The drawing under review shows one solid part. Ordinate dimensions are in mm from its lowest x, y, z. Round coordinates to 2 decimals unless told otherwise and drop trailing zeros. Order: outer loops, then holes, each group sorted by start corner. A loop starts at its lowest first (then second) coordinate and runs counter-clockwise, first axis right, second up. Notation, with made-up numbers: M 78.5,36.25 L 136.5,36.25 A19 ccw 136.5,51.25 Z; hole C 27,-35 d5. An arc over 180 degrees is marked long. Answer as a JSON object with one key per item and string values.
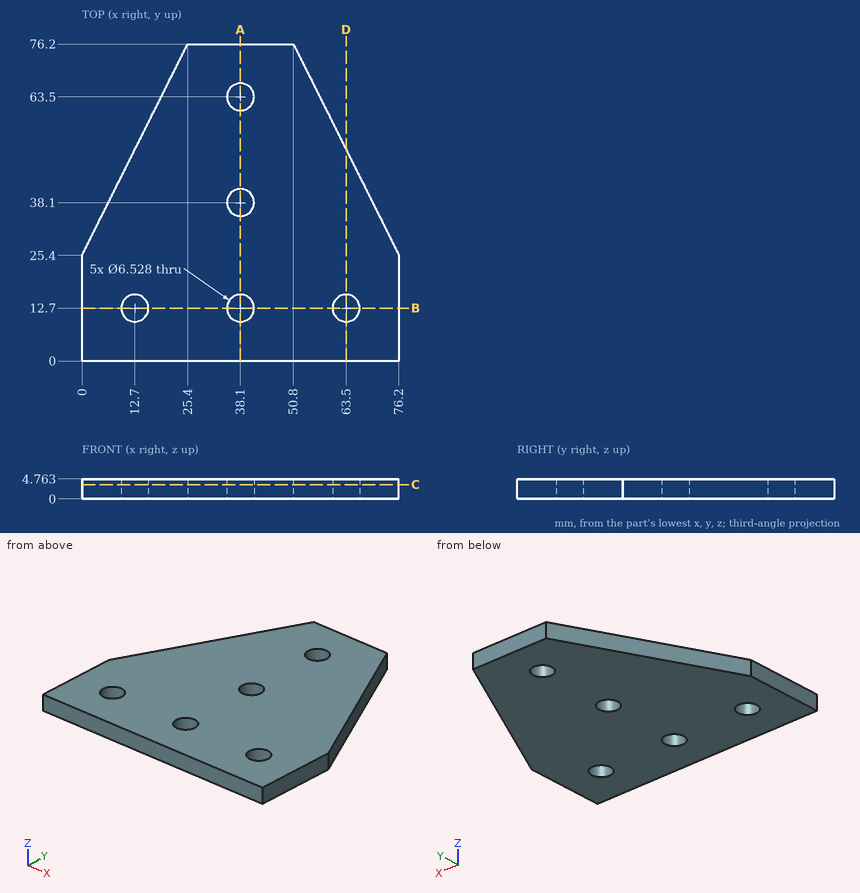
1) Add section A-A on x = 38.1. State the section outline as (y, z) points.
Geometry check:
{"outline": "M 0,0 L 9.44,0 L 9.44,4.76 L 0,4.76 Z; M 15.96,0 L 34.84,0 L 34.84,4.76 L 15.96,4.76 Z; M 41.36,0 L 60.24,0 L 60.24,4.76 L 41.36,4.76 Z; M 66.76,0 L 76.2,0 L 76.2,4.76 L 66.76,4.76 Z"}
2) Insertion check: P1, Ø5, axis at x = 34, y = 13.5, coming from the -Z side; P2, Ø12, axis at x = 67, y = 64.5, coming from the +Z side; P3, Ø1, axis at x = 58.5, z = 1, coming from the +Y side; P4, Ø1, axis at x = 62, z = 1.5, coming from the +Y side. Each pin has a flat end and moves straight along its axis. Give the tip position at first contact, or say it passes through.
Geometry check:
{"P1": "stops at z = 0", "P2": "passes through", "P3": "stops at y = 61.8", "P4": "stops at y = 54.8"}
3) Add section C-C on z = 3.4. State the section outline as (x, y) points.
Geometry check:
{"outline": "M 0,0 L 76.2,0 L 76.2,25.4 L 50.8,76.2 L 25.4,76.2 L 0,25.4 Z; hole C 12.7,12.7 d6.53; hole C 38.1,12.7 d6.53; hole C 38.1,38.1 d6.53; hole C 38.1,63.5 d6.53; hole C 63.5,12.7 d6.53"}
4) Add section D-D on x = 63.5. State the section outline as (y, z) points, and give its area (3 significant figures).
Geometry check:
{"outline": "M 0,0 L 9.44,0 L 9.44,4.76 L 0,4.76 Z; M 15.96,0 L 50.8,0 L 50.8,4.76 L 15.96,4.76 Z", "area": "211 mm²"}
5) For L1, parallel to Y at x = 38.1, z = 1.05; L2, parallel to X at y = 13, z = 3.65; L3, parallel to X at y = 11, z = 3.95 (1 decimal), list the stretches that pass through material, from the lowest coordinate up.
Geometry check:
{"L1": "y = 0 to 9.44, 15.96 to 34.84, 41.36 to 60.24, 66.76 to 76.2", "L2": "x = 0 to 9.45, 15.95 to 34.85, 41.35 to 60.25, 66.75 to 76.2", "L3": "x = 0 to 9.9, 15.5 to 35.3, 40.9 to 60.7, 66.3 to 76.2"}
